```python
from build123d import *

# Parameters (mm, degrees)
SKETCH1_R           = 1.5875
BOSS_EXTRUDE1_DEPTH = 70.0659
SKETCH2_W           = 0.381
SKETCH2_H           = 0.381


with BuildPart() as part:
    # Sketch1 → Boss-Extrude1 (new, symmetric)
    with BuildSketch(Plane(origin=(0, 0, 0), x_dir=(1, 0, 0), z_dir=(0, 1, 0))):
        with Locations(Location((0, 0, 0), (0, 0, 270))):
            Circle(SKETCH1_R)
    extrude(amount=BOSS_EXTRUDE1_DEPTH, both=True)

    # Sketch2 → Cut-Revolve1 (revolve, cut)
    with BuildSketch(Plane.XY, mode=Mode.PRIVATE) as cut_revolve1_sk:
        with Locations((1.397, 58.8137)):
            Rectangle(SKETCH2_W, SKETCH2_H)
        with Locations((1.397, -58.8137)):
            Rectangle(SKETCH2_W, SKETCH2_H)
        with Locations((1.397, 66.6369)):
            Rectangle(SKETCH2_W, SKETCH2_H)
        with Locations((1.397, -66.6369)):
            Rectangle(SKETCH2_W, SKETCH2_H)
    revolve(cut_revolve1_sk.sketch.rotate(Axis((0, -58.6232, 0), (0, 1, 0)), 90), axis=Axis((0, -58.6232, 0), (0, 1, 0)), mode=Mode.SUBTRACT)


solid = part.part
```
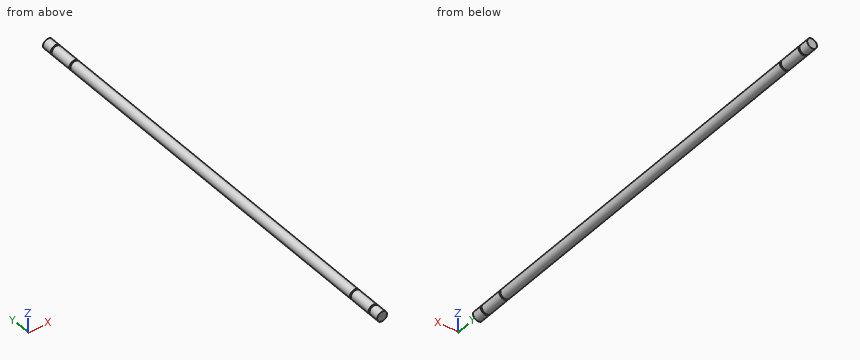
Read the model definition and answer for the solid it produces. Units are mm, in the model's axes. Give positions to 0.01 mm unless a question says otherwise; leave off trailing zeros. Order: outer loops, then holes, each group sorted by start corner. A loop starts at its lowest first (then second) coordinate and runs counter-clockwise, first axis right, second up. Notation, with made-up numbers: (47, 14.25) -> (104, 14.25) arc R31 ccw to (104, 47.25) -> close; hole circle Ø6 at (18, -26). An arc over 180 degrees is marked (long way). One line per item, written item: value. Start each with the question number.
(1) A flat-ended cylindrical pin translates along its axis: P1, Ø1, axis at y = -41, z = -1, coming from the +X side. Find the tip coordinate at first contact, or state that the pin passes through.
(2) Straight lines are drawn through the part: L1, parallel to Y at x = 0.95, z = 1.2; L2, parallel to X at y = 52.5, z = 1.05; L3, parallel to Z at x = 0.2, y = -35.5. For each, find the intervals that lie inside material, in ascending order.
(3) The part is cut by section A-A (y = 42). Determine the outline of the cut face in (x, z) (1 decimal), and give its area (3 significant figures).
Taken from the geometry:
1. P1: x = 1.51
2. L1: -70.07 to -66.83, -66.45 to -59, -58.62 to 58.62, 59 to 66.45, 66.83 to 70.07
2. L2: -1.19 to 1.19
2. L3: -1.57 to 1.57
3. outline: circle Ø3.2 at (0, 0)
3. area: 7.92 mm^2
